Part model, mm, in its own coordinate system. A direction names the side the tool comes from. Give positions to 0.01 mm unless a question says otherwise; leave off trailing zeros. Order: outer loops, then holes, each group sorted by start corner. A loop starts at its lowest first (then second) coordinate and runs counter-clockwise, first axis right, second up. Notation, with made-up numbers: (-18.5, 22) -> (-11.5, 22) arc R19 ccw to (-11.5, 45) -> close; hole circle Ø9 at (47, 50.5). An arc over 180 degrees is marked (long way). Write item = value, one per line. Start each with the question number.
Item 1: Drill centre lines: line 1 along X through (y, z) = (-15, 3.75); line 2 along Z through (x, y) = (1.75, -20); line 3 along Z through (x, y) = (-10.25, -43). Where is each one in solid material? Low to high.
Item 2: Flat gauge pins, fed straight in: P1, Ø10, axis at x = 0, y = -31, coming from the +Z side; P2, Ø3, axis at x = 1.5, z = -6, coming from the -Y side; P3, Ø5, axis at x = -8.5, y = -28, coming from the -Z side. Where does each tip first touch, or does it go through?
Item 3: Band-saw the part on B-B on z = 2.75. Write the cut outline in (x, y), plus the area to 3 significant figures.
Item 4: Band-saw the part on C-C on x = -1.5. Write the cut outline in (y, z), plus the area to 3 significant figures.
Item 5: Pull direction X, two halves, no side cores. Call faces 1 (the face through (11.48, -8.63, 3.52)), 2 (the face through (0, -25, 0)), 3 (the face through (13, -25, 0)), 4 (the face through (-10, -25, 2)): +X half, -X half, draft (parallel to the pull), parting line (faces both ways), or undercut.
Item 6: Tool access for faces 5 (the face through (10, -25, 3)), 6 (the face through (-11, -33, 5)), 7 (the face through (0, -32, -3)): list every direction of +Z, -Z, +X, -X, +Y, -Y with a clear straight run to the whole face (end or side of a thin tool).
Item 7: Band-saw the part on D-D on z = -6. Write the cut outline in (x, y), plus the area to 3 significant figures.
Item 8: Band-saw the part on A-A on y = -30.5. Write the cut outline in (x, z), plus the area to 3 significant figures.
```python
from build123d import *

# Parameters (mm, degrees)
PAD_DEPTH         = 50
POCKET_DEPTH      = 13.001
POCKET_DEPTH_BACK = -13.001


with BuildPart() as part:
    # Sketch → Pad (new body)
    with BuildSketch(Plane.XZ):
        Polygon((-13, 5), (-13, -8), (13, -8), (13, 5), (10, 5), (10, 0), (-10, 0), (-10, 5), align=None)
    extrude(amount=PAD_DEPTH)

    # Sketch001 → Pocket (cut, two sides)
    with BuildSketch(Plane.YZ) as pocket_sk:
        Polygon((-17.013845, 5), (0, 2), (0, 5), align=None)
        Polygon((-50, -3), (-50, -8), (-5, -8), (-13.660254, -3), align=None)
    extrude(amount=-POCKET_DEPTH, mode=Mode.SUBTRACT)
    extrude(pocket_sk.sketch, amount=-POCKET_DEPTH_BACK, mode=Mode.SUBTRACT)


solid = part.part
```
Values found:
q1.line_1 = -13 to -10, 10 to 13
q1.line_2 = -3 to 0
q1.line_3 = -3 to 5
q2.P1 = 0
q2.P2 = -11.06
q2.P3 = -3
q3.outline = (-13, -50) -> (-10, -50) -> (-10, -4.25) -> (-13, -4.25) -> close; (10, -50) -> (13, -50) -> (13, -4.25) -> (10, -4.25) -> close
q3.area = 274 mm^2
q4.outline = (-50, -3) -> (-13.66, -3) -> (-5, -8) -> (0, -8) -> (0, 0) -> (-50, 0) -> close
q4.area = 197 mm^2
q5.face_1 = draft
q5.face_2 = undercut
q5.face_3 = +X half
q5.face_4 = undercut
q6.face_5 = +Z, +Y, -Y
q6.face_6 = +Z, +X, -X, +Y, -Y
q6.face_7 = -Z, +X, -X, -Y
q7.outline = (-13, -8.46) -> (13, -8.46) -> (13, 0) -> (-13, 0) -> close
q7.area = 220 mm^2
q8.outline = (-13, -3) -> (13, -3) -> (13, 5) -> (10, 5) -> (10, 0) -> (-10, 0) -> (-10, 5) -> (-13, 5) -> close
q8.area = 108 mm^2
